Geometry: final body of the model. Coordinates: model frame, mm. A direction names the side the tool comes from. Round coordinates to 2 decimals unless told otherwise and drop trailing zeros. Loops run counter-clockwise (first coordinate to the right, second up) from the corner with the lowest first, then second, coordinate; pieces in that order, holes last. Notation, with made-up numbers: (-13, 71.25) - (28, 71.25) arc R10 ccw to (28, 77.25) - close; hole circle Ø3 at (17, -8.75). An arc over 180 degrees is marked (long way). Return JSON: item names as keys, results as strings. Group by question number.
1. Material intervals for probe 1 along X at (y, z) = (9.15, -60.96); probe 2 along X at (y, z) = (11.15, -60.96); probe 3 along Z at (x, y) = (-4, 9.5), sorted ascending.
2. Section A-A on x = 0. Return loops of the section in (y, z).
3. First-contact query: pin 1 Ø2.5 at (x, z) = (0, 0) entering from +Y; pin 2 Ø18.5 at (x, z) = (0, -60.96) entering from -Y; pin 3 Ø10 at (x, z) = (-5.5, -53) entering from -Y; pin 4 Ø3 at (x, y) = (3, 2) entering from +Z. Flat tips, straight axial feed; report the tip coordinate or a pass-through.
4. Set-up query: faces 1 (the face through (0.371, 5.916, 16.846)), 2 (the face through (8, 10.5, -59)), 3 (the face through (0, 3, -40.64)). Return all of +Z, -Z, +X, -X, +Y, -Y with unobstructed straight access to the full face (end or side cutting, diameter ignored); none if empty.
5. Section B-B on z = -68. Return loops of the section in (x, y), and give its area (3 significant figures).
6. Draft query along Z for faces 4 (the face through (-0.371, 8.958, -77.806)), 5 (the face through (0, 12, -30)), 6 (the face through (0.46, 8.22, -71.45)). Return one class per face: +Z half, -Z half, draft (parallel to the pull), parting line (faces both ways), or undercut.
7. Section C-C on x = 4.5. Return loops of the section in (y, z).
from build123d import *

# Parameters (mm, degrees)
SKETCH1_R           = 10.499999955
SKETCH1_R_2         = 2
BOSS_EXTRUDE1_DEPTH = 12
SKETCH2_R           = 10.499999955
CUT_EXTRUDE1_DEPTH  = 6
BOSS_EXTRUDE2_START = -1.5
SKETCH3_R           = 10.499999955
SKETCH3_R_2         = 8
BOSS_EXTRUDE2_DEPTH = 1.5


with BuildPart() as part:
    # Sketch1 → Boss-Extrude1 (new body)
    with BuildSketch(Plane(origin=(0, 0, 0), x_dir=(1, 0, 0), z_dir=(0, 1, 0))):
        with BuildLine():
            Line((-16.85, 0), (-16.85, 60.96))
            ThreePointArc((-16.85, 60.96), (0, 77.81), (16.85, 60.96))
            Line((16.85, 60.96), (16.85, 0))
            ThreePointArc((16.85, 0), (0, -16.85), (-16.85, 0))
        make_face()
        with Locations(Location((0, 60.96, 0), (0, 0, 270))):
            Circle(SKETCH1_R, mode=Mode.SUBTRACT)
        with Locations(Location((-8, 0, 0), (0, 0, 270))):
            Circle(SKETCH1_R_2, mode=Mode.SUBTRACT)
        with Locations(Location((8, 0, 0), (0, 0, 270))):
            Circle(SKETCH1_R_2, mode=Mode.SUBTRACT)
        with Locations(Location((0, 0, 0), (0, 0, 270))):
            Circle(SKETCH1_R_2, mode=Mode.SUBTRACT)
    extrude(amount=BOSS_EXTRUDE1_DEPTH)

    # Sketch2 → Cut-Extrude1 (cut)
    with BuildSketch(Plane.XZ):
        with BuildLine():
            Line((-16.85, -40.64), (-16.85, -60.96))
            ThreePointArc((-16.85, -60.96), (0, -77.81), (16.85, -60.96))
            Line((16.85, -60.96), (16.85, -40.64))
            Line((16.85, -40.64), (-16.85, -40.64))
        make_face()
        with Locations(Location((0, -60.96, 0), (0, 0, 270))):
            Circle(SKETCH2_R, mode=Mode.SUBTRACT)
    extrude(amount=-CUT_EXTRUDE1_DEPTH, mode=Mode.SUBTRACT)

    # Sketch3 → Boss-Extrude2 (add)
    with BuildSketch(Plane(origin=(0, 12, 0), x_dir=(1, 0, 0), z_dir=(0, 1, 0)).offset(BOSS_EXTRUDE2_START)):
        with Locations(Location((0, 60.96, 0), (0, 0, 90))):
            Circle(SKETCH3_R)
        with Locations(Location((0, 60.96, 0), (0, 0, 270))):
            Circle(SKETCH3_R_2, mode=Mode.SUBTRACT)
    extrude(amount=BOSS_EXTRUDE2_DEPTH)


solid = part.part
Taken from the geometry:
{
 "1": {"probe 1": "-16.85 to -10.5, 10.5 to 16.85", "probe 2": "-16.85 to -8, 8 to 16.85", "probe 3": "-77.33 to -70.67, -51.25 to 16.37"},
 "2": {"outline": "(0, -40.64) - (6, -40.64) - (6, -50.46) - (10.5, -50.46) - (10.5, -52.96) - (12, -52.96) - (12, -2) - (0, -2) - close; (0, 2) - (12, 2) - (12, 16.85) - (0, 16.85) - close; (6, -77.81) - (12, -77.81) - (12, -68.96) - (10.5, -68.96) - (10.5, -71.46) - (6, -71.46) - close"},
 "3": {"pin 1": "through", "pin 2": "y = 10.5", "pin 3": "y = 6", "pin 4": "z = 16.78"},
 "4": {"face 1": "+Z, +Y, -Y", "face 2": "-Y", "face 3": "-Z, +X, -X, -Y"},
 "5": {"outline": "(-15.31, 6) - (-7.79, 6) - (-7.79, 10.5) - (-3.8, 10.5) - (-3.8, 12) - (-15.31, 12) - close; (3.8, 10.5) - (7.79, 10.5) - (7.79, 6) - (15.31, 6) - (15.31, 12) - (3.8, 12) - close", "area": "102 mm2"},
 "6": {"face 4": "-Z half", "face 5": "draft", "face 6": "undercut"},
 "7": {"outline": "(0, -40.64) - (6, -40.64) - (6, -51.47) - (10.5, -51.47) - (10.5, -54.35) - (12, -54.35) - (12, 16.24) - (0, 16.24) - close; (6, -77.2) - (12, -77.2) - (12, -67.57) - (10.5, -67.57) - (10.5, -70.45) - (6, -70.45) - close"}
}
